from build123d import *

# Parameters (mm, degrees)
ESQUISSE1_R    = 15
BASE_DEPTH     = 10
ESQUISSE2_R    = 2.5
VIDE_VIS_DEPTH = 185.746447868
CONGE_CABLE_R  = 5


with BuildPart() as part:
    # Esquisse1 → BASE (new body)
    with BuildSketch(Plane(origin=(0, 0, 0), x_dir=(1, 0, 0), z_dir=(0, 1, 0))):
        Polygon((-82.5, 77.5), (-72.5, 77.5), (-72.5, 67.5), (-82.5, 67.5), (-82.5, -2.5), (-72.5, -2.5), (-72.5, -12.5), (-82.5, -12.5), (-82.5, -82.5), (82.5, -82.5), (82.5, -12.5), (72.5, -12.5), (72.5, -2.5), (82.5, -2.5), (82.5, 67.5), (72.5, 67.5), (72.5, 77.5), (82.5, 77.5), (82.5, 82.5), (-82.5, 82.5), align=None)
        with Locations(Location((0, -0.648107225, 0), (0, 0, 270))):
            Circle(ESQUISSE1_R, mode=Mode.SUBTRACT)
    extrude(amount=BASE_DEPTH)

    # Esquisse2 → VIDE VIS (cut, through all)
    with BuildSketch(Plane(origin=(0, 0, -82.5), x_dir=(-1, 0, 0), z_dir=(0, 0, -1))):
        with Locations((-77.5, 5)):
            Circle(ESQUISSE2_R)
        with Locations(Location((77.5, 5, 0), (0, 0, 180))):
            Circle(ESQUISSE2_R)
    extrude(amount=-VIDE_VIS_DEPTH, mode=Mode.SUBTRACT)

    # CONGE CABLE
    conge_cable_edges = [part.edges().sort_by_distance(p)[0] for p in [
        (0, 0, -14.351892775),
        (0, 10, -14.351892775),
    ]]
    fillet(conge_cable_edges, radius=CONGE_CABLE_R - 0.0001)  # a hair under: the kernel refuses the full size


solid = part.part
Model file for the job. Use its own axes, mm. A direction names the side the tool comes from. Give positions to 0.01 mm unless a question says otherwise; leave off trailing zeros. Loops run counter-clockwise (first coordinate to the right, second up) from the corner with the lowest first, then second, coordinate; pieces in that order, holes last.
Item 1: Slice it at D-D (z = -4). Give the number of separate pieces and of enclosed holes in the cut face, plus the area to 3 significant figures.
Check values:
separate pieces: 2
enclosed holes: 2
area: 1,300 mm2
Item 2: Drop flat-ended pins along their axis: P1, Ø4, axis at x = 77.5, y = 5, coming from the -Z side; P2, Ø3, axis at y = 6.5, z = 6, coming from the -X side; P3, Ø5, axis at y = 5.5, z = 6, coming from the +X side. Give the stop position or say it passes through.
Check values:
P1: passes through
P2: stops at x = -72.5
P3: stops at x = 72.5
Item 3: Mould opens along Y. For faces 1 (the face through (-80, 5, -80)), 2 (the face through (-1.2, 10, -19.5)), 3 (the face through (-75, 4, -67.5)), 4 (the face through (80, 5, -33)) say: +Y half, -Y half, draft (parallel to the pull), parting line (faces both ways), or undercut.
Check values:
face 1: undercut
face 2: +Y half
face 3: draft
face 4: undercut
Item 4: Slice it at B-B (x = 77.5). Write the cut outline in (y, z).
Check values:
outline: (0, -82.5) - (2.5, -82.5) - (2.5, -77.5) - (0, -77.5) - close; (0, -67.5) - (2.5, -67.5) - (2.5, 2.5) - (0, 2.5) - close; (0, 12.5) - (2.5, 12.5) - (2.5, 82.5) - (0, 82.5) - close; (7.5, -82.5) - (10, -82.5) - (10, -77.5) - (7.5, -77.5) - close; (7.5, -67.5) - (10, -67.5) - (10, 2.5) - (7.5, 2.5) - close; (7.5, 12.5) - (10, 12.5) - (10, 82.5) - (7.5, 82.5) - close
Item 5: Slice it at C-C (z = 51). Write the cut outline in (x, y), plus the area to 3 significant figures.
Check values:
outline: (-82.5, 0) - (82.5, 0) - (82.5, 10) - (-82.5, 10) - close; hole circle Ø5 at (-77.5, 5); hole circle Ø5 at (77.5, 5)
area: 1,610 mm2
Item 6: Which spindle directions (+Z, -Z, +X, -X, +Y, -Y) get a long thin tool onto all of the face, cutting with end or side? Do faces 5 (the face through (72.5, 5, -72)), 6 (the face through (-75, 4, 12.5)), 7 (the face through (1, 5, -82.5)). Say none if no direction does.
Check values:
face 5: +X, +Y, -Y
face 6: -X, +Y, -Y
face 7: -Z, +X, -X, +Y, -Y
Item 7: Drill centre lines: line 1 along Z through (x, y) = (75, 8.5); line 2 along X through (y, z) = (3.5, -52.5); line 3 along X through (y, z) = (5.5, 56.5). Where is each one in solid material? Low to high.
Check values:
line 1: z = -82.5 to -77.5, -67.5 to 2.5, 12.5 to 82.5
line 2: x = -82.5 to -79.5, -75.5 to 75.5, 79.5 to 82.5
line 3: x = -82.5 to -79.95, -75.05 to 75.05, 79.95 to 82.5
